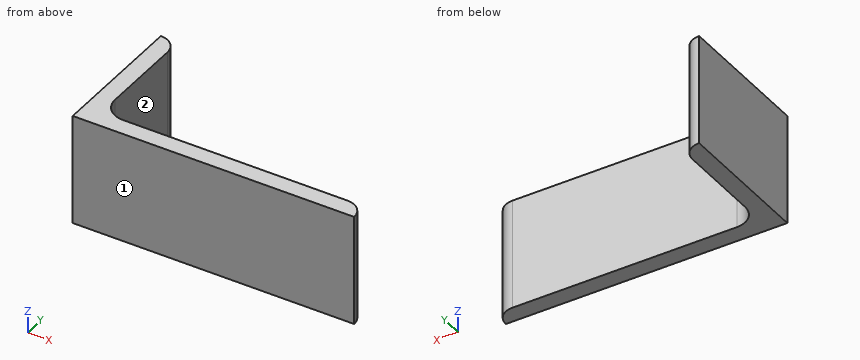
```python
from build123d import *

# Parameters (mm, degrees)
HIERRO_ANGULAR_3_X_2_X_0_25_1_DEPTH = 40


with BuildPart() as part:
    # Sketch1 → Hierro angular 3 X 2 X 0.25(1) (new body)
    with BuildSketch(Plane.YX):
        with BuildLine():
            Line((0, 0), (0, 102))
            Line((0, 102), (0.00508, 102))
            ThreePointArc((0.00508, 102), (4.491615958, 100.141615958), (6.35, 95.65508))
            Line((6.35, 95.65508), (6.35, 14.2875))
            ThreePointArc((6.35, 14.2875), (8.674839924, 8.674839924), (14.2875, 6.35))
            Line((14.2875, 6.35), (44.45508, 6.35))
            ThreePointArc((44.45508, 6.35), (48.941615958, 4.491615958), (50.8, 0.00508))
            Line((50.8, 0.00508), (50.8, 0))
            Line((50.8, 0), (0, 0))
        make_face()
    extrude(amount=HIERRO_ANGULAR_3_X_2_X_0_25_1_DEPTH)


solid = part.part
```
Work out the finished part from the listing and answer in its coordinate system (mm). Face numbers are marked on the shaded views. A direction names the side the tool comes from. Round coordinates to 2 decimals unless told otherwise and drop trailing zeros. Write each loop counter-clockwise with the first axis right and the second up, starting at its lowest first coordinate (ties: lowest second). Pieces come first, ordered by that corner, then holes. Notation, with made-up numbers: (54.25, 14) -> (59.25, 14) arc R31 cw to (59.25, 40) -> close; hole circle Ø5 at (-32, -16.75). An arc over 180 degrees is marked (long way). Write each question's results on one line, items separated by ' | '.
1) Consider line 1 along Y through (x, z) = (84.5, -12); line 2 along Y through (x, z) = (5.5, -20.5). Determine where each line is inside the solid, lowest interval first. Write a range as [from, to].
Findings:
line 1: y = [0, 6.35] | line 2: y = [0, 47.63]
2) Flat-ended cylindrical pins translate along their axes: pin 1 (2 mm diameter, centred on x = 45.5, z = -31, fed in from +Y); pin 2 (8 mm diameter, centred on y = 11, z = -11.5, fed in from +X); pin 3 (15 mm diameter, centred on y = 23, z = -23.5, fed in from +X). Find the tip coordinate at first contact, or state that the pin passes through.
Findings:
pin 1: stops at y = 6.35 | pin 2: stops at x = 11.14 | pin 3: stops at x = 6.35
3) Which of the six approach directions +Z, -Z, +X, -X, +Y, -Y give full straight-line access (tool end or side, diameter ignored) to the marked faces 1 and 2?
Findings:
face 1: +Z, -Z, +X, -X, -Y | face 2: +Z, -Z, +X, +Y
4) The part is cut by section B-B (y = 21). Write down the section's boundary in (x, z).
Findings:
outline: (0, -40) -> (6.35, -40) -> (6.35, 0) -> (0, 0) -> close
